The listing builds one solid part. Answer for the finished solid, in the listing's coordinates (mm). Face numbers are marked on the shaded views. Round coordinates to 2 decimals unless told otherwise and drop trailing zeros. Order: outer loops, then holes, each group sorted by start corner. A loop starts at its lowest first (then second) coordinate and runs counter-clockwise, first axis right, second up. Notation, with made-up numbers: (70.25, -15) -> (122.25, -15) arc R22 cw to (122.25, 11) -> close; hole circle Ø6 at (8, 56.25). An arc over 180 degrees is marked (long way). Return JSON: item names as keys, results as strings. Group by question number.
(1) The part is cut by section B-B (x = 0). Determine the outline of the cut face in (y, z), plus the area to 3 significant figures.
(2) The part is cut by section A-A (z = 23). Determine the outline of the cut face in (x, y), plus the area to 3 significant figures.
(3) Determine the mould class of the marked faces 1, 2, 3 and 4 for opening direction Y: +Y half, -Y half, draft (parallel to the pull), parting line (faces both ways), or undercut.
(4) Consider line 1 (Y direction, x = 0, z = 17.5); line 2 (X direction, y = -7, z = 6); line 3 (Z direction, x = -7, y = 0.5). Determine where each line is inside the solid, lowest interval first. Write a range as [from, to].
(5) Each of these flat-tipped pins is pushed along its axis until it touches: pin 1 (4 mm diameter, centred on x = 5.5, y = 0, fed in from -Z); pin 2 (6 mm diameter, centred on y = 8, z = 17.5, fed in from +X). Where does it stop, or does it pass through?
(6) The part is cut by section D-D (x = -8). Determine the outline of the cut face in (y, z), plus the area to 3 significant figures.
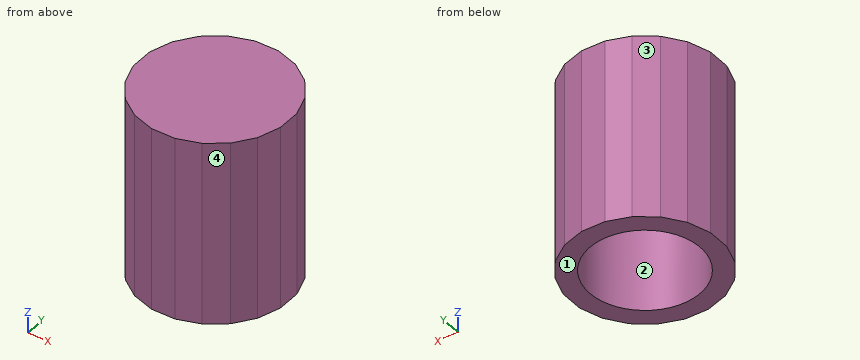
from build123d import *

# Parameters (mm, degrees)
F0_R     = 7.62
F1_DEPTH = 25.4
F2_DEPTH = 23.486745


with BuildPart() as f1:
    # F0 (on Top) → F1 (new body)
    with BuildSketch(Plane.XY):
        Polygon((1.609186, 10.16), (-1.609186, 10.16), (-4.670039, 9.165468), (-7.273757, 7.273757), (-9.165468, 4.670039), (-10.16, 1.609186), (-10.16, -1.609186), (-9.165468, -4.670039), (-7.273757, -7.273757), (-4.670039, -9.165468), (-1.609186, -10.16), (1.609186, -10.16), (4.670039, -9.165468), (7.273757, -7.273757), (9.165468, -4.670039), (10.16, -1.609186), (10.16, 1.609186), (9.165468, 4.670039), (7.273757, 7.273757), (4.670039, 9.165468), align=None)
        Circle(F0_R, mode=Mode.SUBTRACT)
        Circle(F0_R)
    extrude(amount=F1_DEPTH)

    # F0 (on Top) → F2 (cut)
    with BuildSketch(Plane.XY):
        Circle(F0_R)
    extrude(amount=F2_DEPTH, mode=Mode.SUBTRACT)


solid = f1.part
Answer below:
{
 "1": {"outline": "(-10.16, 0) -> (-7.62, 0) -> (-7.62, 23.49) -> (7.62, 23.49) -> (7.62, 0) -> (10.16, 0) -> (10.16, 25.4) -> (-10.16, 25.4) -> close", "area": "158 mm²"},
 "2": {"outline": "(-10.16, -1.61) -> (-9.17, -4.67) -> (-7.27, -7.27) -> (-4.67, -9.17) -> (-1.61, -10.16) -> (1.61, -10.16) -> (4.67, -9.17) -> (7.27, -7.27) -> (9.17, -4.67) -> (10.16, -1.61) -> (10.16, 1.61) -> (9.17, 4.67) -> (7.27, 7.27) -> (4.67, 9.17) -> (1.61, 10.16) -> (-1.61, 10.16) -> (-4.67, 9.17) -> (-7.27, 7.27) -> (-9.17, 4.67) -> (-10.16, 1.61) -> close; hole circle Ø15.24 at (0, 0)", "area": "145 mm²"},
 "3": {"face 1": "draft", "face 2": "undercut", "face 3": "+Y half", "face 4": "-Y half"},
 "4": {"line 1": "y = [-10.16, -7.62], [7.62, 10.16]", "line 2": "x = [-7.47, -3.01], [3.01, 7.47]", "line 3": "z = [23.49, 25.4]"},
 "5": {"pin 1": "stops at z = 23.49", "pin 2": "stops at x = 8.93"},
 "6": {"outline": "(-6.27, 0) -> (6.27, 0) -> (6.27, 25.4) -> (-6.27, 25.4) -> close", "area": "319 mm²"}
}
